Input: part model. Units: mm. Frame: model coordinates. Coordinates: 2 decimals unless noted, no trailing zeros. Order: outer loops, then holes, each group sorted by start corner. A loop starts at its lowest first (then second) coordinate and runs counter-clockwise, first axis right, second up. Notation, with made-up numbers: (-28.5, -36) -> (3.5, -36) arc R14 ccw to (3.5, -27) -> close; hole circle Ø8 at (41.5, 48). An arc over 180 degrees is marked (long way). Write each question's results on one line, items separated by ' | '.
```python
from build123d import *

# Parameters (mm, degrees)
SKETCH1_W               = 50
SKETCH1_H               = 20
BOSS_EXTRUDE1_DEPTH     = 125
SKETCH3_W               = 50
SKETCH3_H               = 250
BOSS_EXTRUDE2_DEPTH     = 5
CUT_EXTRUDE1_DEPTH      = 130.903810568
CUT_EXTRUDE1_DEPTH_BACK = 10
SKETCH2_R               = 2.5
FILLET1_R               = 2


with BuildPart() as part:
    # Sketch1 → Boss-Extrude1 (new, symmetric)
    with BuildSketch(Plane.XY):
        Rectangle(SKETCH1_W, SKETCH1_H)
    extrude(amount=BOSS_EXTRUDE1_DEPTH, both=True)

    # Sketch3 → Boss-Extrude2 (add)
    with BuildSketch(Plane(origin=(0, 10, 0), x_dir=(1, 0, 0), z_dir=(0, 1, 0))):
        Rectangle(SKETCH3_W, SKETCH3_H)
    extrude(amount=BOSS_EXTRUDE2_DEPTH)

    # Sketch2 → Cut-Extrude1 (cut, two sides: drawn at the far end of the back side and taken through both)
    with BuildSketch(Plane(origin=(0, 15, 0), x_dir=(1, 0, 0), z_dir=(0, 1, 0)).offset(-CUT_EXTRUDE1_DEPTH_BACK)):
        with Locations(Location((0, 115, 0), (0, 0, 90))):
            Circle(SKETCH2_R)
    extrude(amount=CUT_EXTRUDE1_DEPTH + CUT_EXTRUDE1_DEPTH_BACK, mode=Mode.SUBTRACT)

    # Fillet1
    fillet1_edges = [part.edges().sort_by_distance(p)[0] for p in [
        (-25, 15, 0),
        (25, 15, 0),
    ]]
    fillet(fillet1_edges, radius=FILLET1_R)


solid = part.part
```
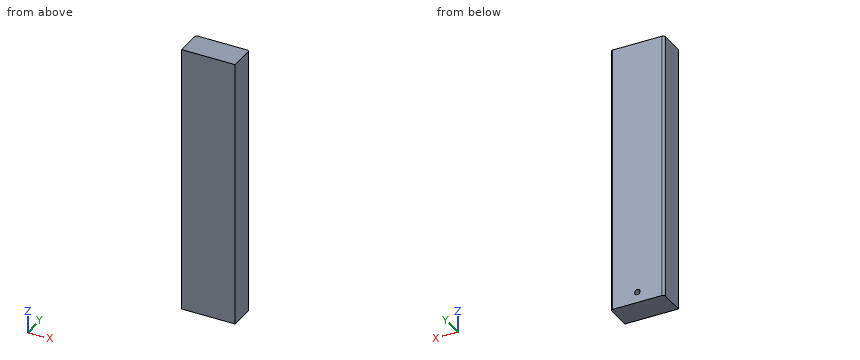
(1) Cut plane A-A, the plane z = -115. Return loops of the section in (x, y), plus the area to 3 significant figures.
Return value:
outline: (-25, -10) -> (25, -10) -> (25, 13) arc R2 ccw to (23, 15) -> (2.5, 15) -> (2.5, 5) -> (-2.5, 5) -> (-2.5, 15) -> (-23, 15) arc R2 ccw to (-25, 13) -> close | area: 1,200 mm2
(2) Line query: line 1 along X through (y, z) = (11, -115); line 2 along X through (y, z) = (13.5, 53). Output: solid intervals per line, ascending. Write a range as from..to.
Return value:
line 1: -25..-2.5, 2.5..25 | line 2: -24.94..24.94
(3) Pin query (flat end, axial travel): P1, Ø1.5, axis at x = -1, z = -114.5, coming from the +Y side. Return the tip coordinate at first contact, or that it passes through.
Return value:
P1: y = 5
